Geometry: see drawing. Coordinates: mm, zero at the bounding-box minimum. A direction names the side the tool comes from. Give positions to 0.01 mm unless a question says otherwise; leave off trailing zeros. Write each loop counter-clockwise with the first axis right and the second up, starting at its lowest first coordinate (ties: lowest second). Pieces come first, ordered by that corner, then holes. Notation, with made-up numbers: (89.25, -3) - (97.25, -3) arc R19 ccw to (97.25, 7) - close; hole circle Ø11 at (51, -27). An arc over 180 degrees is marked (long way). Answer as CSV lines item,"result". Start each with the question number.
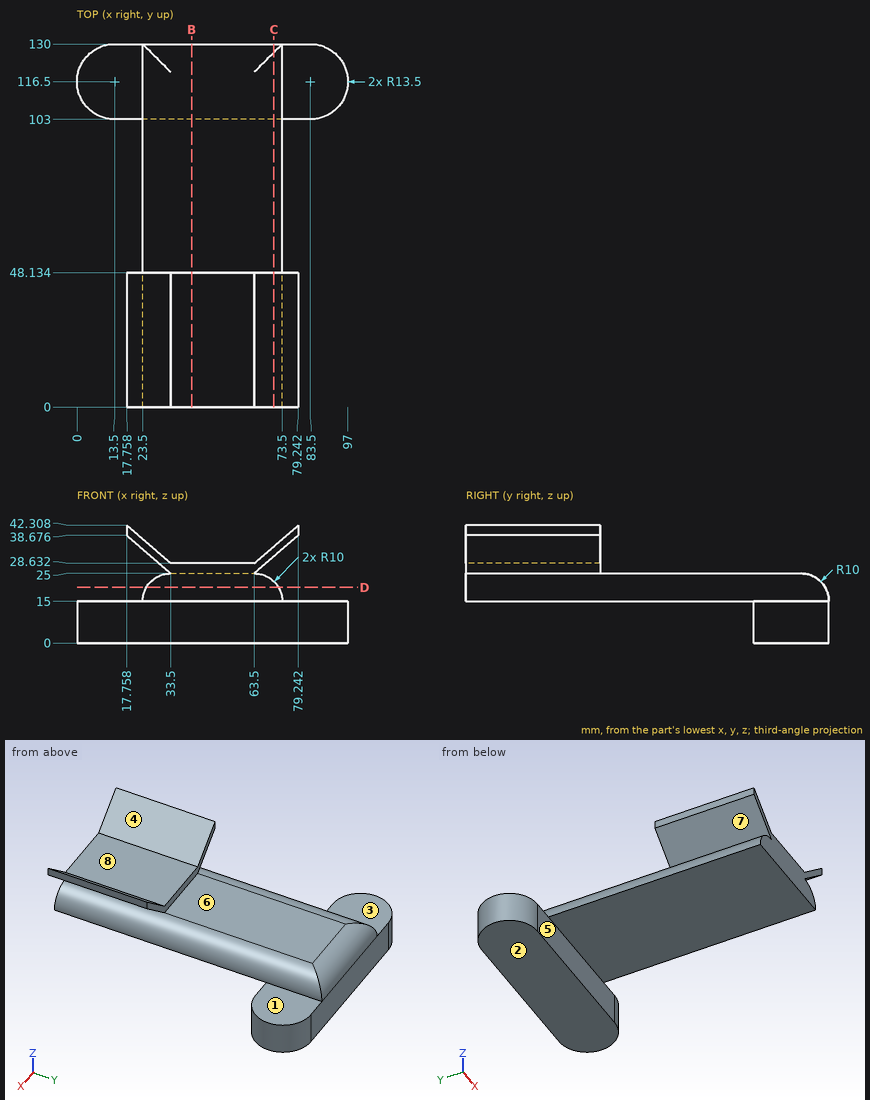
1) Contact query for flat-ended pins moving along their axis: P1, Ø10, axis at y = 76.5, z = 33.5, coming from the -X side; P2, Ø25, axis at x = 38, y = 60, coming from the -Z side; P3, Ø12, axis at x = 10, y = 123, coming from the +Z side; P4, Ø3, axis at y = 26, z = 40, coming from the +X side. Output: stop coordinate, or through.
2) Cut plane D-D on z = 20. Output: boundary loops of the cut face in (x, y), and give its area (3 significant figures).
3) Reachability of the marked faces 1, 2, 3, 4 and 5 from +Z, -Z, +X, -X, +Y, -Y: full face, straight path, thin tool, end or side. Return the list, or none.
4) Cut plane C-C on x = 70.5. Output: boundary loops of the cut face in (y, z), and give its area (3 significant figures).
5) Pull-direction query (X, two-part tool) for the marked faces 6, 7 and 8; classes: +X half, -X half, draft (parallel to the pull), parting line (faces both ways), or undercut.
6) Material intervals for line 1 (Y direction, x = 50, z = 15.5); line 2 (Z direction, x = 15.5, y = 117); line 3 (X direction, y = 17.5, z = 32), sorted ascending. Write a range as from..to.
7) Cut plane B-B on x = 41. Output: boundary loops of the cut face in (y, z).
Numbers:
1,P1,"passes through"
1,P2,"stops at z = 15"
1,P3,"stops at z = 15"
1,P4,"stops at x = 79.24"
2,outline,"(24.84, 0) - (72.16, 0) - (72.16, 128.66) - (24.84, 128.66) - close"
2,area,"6,090 mm²"
3,face 1,"+Z, +X, +Y, -Y"
3,face 2,"-Z, +X, -X, +Y, -Y"
3,face 3,"+Z, -X, +Y, -Y"
3,face 4,"+Z, +Y, -Y"
3,face 5,"-Z, +X, -X, -Y"
4,outline,"(0, 15) - (103, 15) - (103, 0) - (130, 0) - (130, 15) arc R10 ccw to (127, 22.14) - (0, 22.14) - close; (0, 31.08) - (48.13, 31.08) - (48.13, 34.71) - (0, 34.71) - close"
4,area,"1,500 mm²"
5,face 6,"draft"
5,face 7,"-X half"
5,face 8,"undercut"
6,line 1,"y = 0..129.99"
6,line 2,"z = 0..15"
6,line 3,"x = 25.44..29.62, 67.38..71.56"
7,outline,"(0, 15) - (103, 15) - (103, 0) - (130, 0) - (130, 15) arc R10 ccw to (120, 25) - (48.13, 25) - (48.13, 28.63) - (0, 28.63) - close"
